```python
from build123d import *

# Parameters (mm, degrees)
SKETCH1_R           = 1.55
BOSS_EXTRUDE1_DEPTH = 3
BOSS_EXTRUDE2_DEPTH = 10
CUT_EXTRUDE1_REACH  = 18.249
SKETCH3_RX          = 1.55
SKETCH3_RY          = 1.549991194
CHAMFER1_SIZE       = 1
CHAMFER2_SIZE       = 1
CHAMFER3_SIZE       = 1


with BuildPart() as part:
    # Sketch1 → Boss-Extrude1 (new body)
    with BuildSketch(Plane.XY):
        with BuildLine():
            Line((9.241088209, 28.022032198), (2.675653796, 31.16807272))
            Line((2.675653796, 31.16807272), (-1.142729479, 32.359688918))
            Line((-1.142729479, 32.359688918), (-4.151560379, 22.718271148))
            Line((-4.151560379, 22.718271148), (5.91942551, 19.575383426))
            ThreePointArc((5.91942551, 19.575383426), (11.509238759, 22.253627274), (9.241088209, 28.022032198))
        make_face()
        with Locations((7.274888935, 23.918794401)):
            Circle(SKETCH1_R, mode=Mode.SUBTRACT)
    extrude(amount=BOSS_EXTRUDE1_DEPTH)

    # Sketch2 → Boss-Extrude2 (add)
    with BuildSketch(Plane.XY.offset(3)):
        Polygon((-1.142729479, 32.359688918), (-4.151560379, 22.718271148), (-0.333177104, 21.52665495), (2.675653796, 31.16807272), align=None)
    extrude(amount=BOSS_EXTRUDE2_DEPTH)

    # Sketch3 → Cut-Extrude1 (cut, up to next)
    with BuildSketch(Plane(origin=(-10.243698191, 3.196786653, 0), x_dir=(0, 0, 1), z_dir=(-0.954595819, 0.297904049, 0)), mode=Mode.PRIVATE) as cut_extrude1_sk1:
        with Locations(Location((8.05588909, 25.857711156), (0, 0, -179.999999999))):
            Ellipse(SKETCH3_RX, SKETCH3_RY)
    cut_extrude1_tool1 = extrude(cut_extrude1_sk1.sketch, amount=-CUT_EXTRUDE1_REACH, mode=Mode.PRIVATE) & part.part
    add(cut_extrude1_tool1.solids().sort_by_distance((-2.540581, 27.88045, 8.055889))[0], mode=Mode.SUBTRACT)

    # Chamfer1
    chamfer1_edges = [part.edges().sort_by_distance(p)[0] for p in [
        (-2.242368741, 22.122463049, 13),
        (0.766462159, 31.763880819, 13),
    ]]
    chamfer(chamfer1_edges, length=CHAMFER1_SIZE)

    # Chamfer2
    chamfer2_edges = [part.edges().sort_by_distance(p)[0] for p in [
        (1.171238346, 26.347363835, 3),
    ]]
    chamfer(chamfer2_edges, length=CHAMFER2_SIZE)

    # Chamfer3
    chamfer3_edges = [part.edges().sort_by_distance(p)[0] for p in [
        (-2.647144929, 27.538980033, 0),
    ]]
    chamfer(chamfer3_edges, length=CHAMFER3_SIZE)


solid = part.part
```
Verification items for the finished model (mm, model axes). A direction names the side the tool comes from. Round coordinates to 2 decimals unless told otherwise and drop trailing zeros. Loops run counter-clockwise (first coordinate to the right, second up) from the corner with the lowest first, then second, coordinate; pieces in that order, holes last. Notation, with made-up numbers: (50, -28) -> (62, -28) arc R28 ccw to (62, 6) -> close; hole circle Ø7 at (-15.75, 79). An arc over 180 degrees is marked (long way). Answer as a JSON object with one key per item and string values.
Q1. Section check C-C (y = 22). Record the boundary of the cut face in (x, z).
Data:
{"outline": "(-1.85, 0) -> (11.4, 0) -> (11.4, 3) -> (0.86, 3) -> (-0.19, 4) -> (-0.19, 12.5) -> (-1.85, 12) -> close"}
Q2. Section check D-D (x = 2). Record the boundary of the cut face in (y, z), then the cut area to 3 significant figures.
Data:
{"outline": "(20.8, 0) -> (31.38, 0) -> (31.38, 12) -> (30.33, 13) -> (29, 13) -> (29, 4) -> (25.65, 3) -> (20.8, 3) -> close", "area": "56.7 mm2"}
Q3. Draft check along Y on faces 1 (the flat face through (4, 26, 0)), 2 (the cylindrical face through (7.073, 25.456, 1.479)), 3 (the flat face through (-2.16, 27.46, 0.51)). Enter one of: pulls with the +Y half, pulls with the -Y half, needs draft (parallel to the pull), parting line crosses it, or undercut.
Data:
{"face 1": "needs draft", "face 2": "undercut", "face 3": "pulls with the +Y half"}
Q4. Section check B-B (z = 10.5). Record the boundary of the cut face in (x, y), then the cut area to 3 significant figures.
Data:
{"outline": "(-4.15, 22.72) -> (-0.33, 21.53) -> (2.68, 31.17) -> (-1.14, 32.36) -> close", "area": "40.4 mm2"}
Q5. Scan lines: line 1 (Z direction, x = 2.25, y = 25.75); line 2 (X direction, y = 30.25, z = 9.75); line 3 (X direction, y = 26.25, z = 9.75). Record each from-to range of solid material in increasing order. Write a range as from..to.
Data:
{"line 1": "z = 0..3", "line 2": "x = -1.8..2.39", "line 3": "x = -3.05..1.14"}
Q6. Go/stop test with flat-tipped pins: P1, Ø1, axis at y = 29.5, z = 1.5, coming from the -X side; P2, Ø6, axis at x = -2, z = 2, coming from the -Y side; P3, Ø3, axis at y = 24.5, z = 6, coming from the -X side; P4, Ø3, axis at x = 5, z = 6.5, coming from the +Y side. Record where each tip stops, or that it passes through.
Data:
{"P1": "stops at x = -2.19", "P2": "stops at y = 21.11", "P3": "stops at x = -4.06", "P4": "passes through"}
Q7. Access from +Z, -Z, +X, -X, +Y, -Y to the whole of each face (thin tool, end or side, straight path). Record for faces 4 (the flat face through (-2.96, 26.54, 6.92)), 5 (the flat face through (0.816, 25.209, 9.437)).
Data:
{"face 4": "+Z, -Z, -X, +Y", "face 5": "+Z, +X, -Y"}
Q8. Section check A-A (x = 7.75). Record the boundary of the cut face in (y, z).
Data:
{"outline": "(19.39, 0) -> (22.44, 0) -> (22.44, 3) -> (19.39, 3) -> close; (25.39, 0) -> (28.74, 0) -> (28.74, 3) -> (25.39, 3) -> close"}
